CAD build for the part. Positions are in the model's coordinates, mm. A direction names the side the tool comes from. Give positions to 0.01 mm unless a question says otherwise; leave off trailing zeros. Loops run counter-clockwise (first coordinate to the right, second up) from the corner with the lowest first, then second, coordinate; pieces in that order, holes last. Notation, with made-up numbers: M 38,-18 L 65,-18 A27 ccw 65,7 Z; hole C 19.25,6 d6. An arc over 180 degrees is marked long. Answer as CSV lines item,"result".
```python
from build123d import *

# Parameters (mm, degrees)
BOSS_EXTRUDE1_DEPTH = 2.5
CUT_EXTRUDE1_DEPTH  = 2.5
SKETCH7_R           = 1.5
CUT_EXTRUDE3_DEPTH  = 2.5
SKETCH10_R          = 2.075
CUT_EXTRUDE6_DEPTH  = 2.5


with BuildPart() as part:
    # Sketch1 → Boss-Extrude1 (new body)
    with BuildSketch(Plane(origin=(0, 0, 0), x_dir=(1, 0, 0), z_dir=(0, 1, 0))):
        Polygon((0, 23.132168933), (-13.596747752, 18.714317784), (-22, 7.148233317), (-22, -7.148233317), (-13.596747752, -18.714317784), (0, -23.132168933), (13.596747752, -18.714317784), (22, -7.148233317), (22, 7.148233317), (13.596747752, 18.714317784), align=None)
    extrude(amount=BOSS_EXTRUDE1_DEPTH)

    # Sketch2 → Cut-Extrude1 (cut)
    with BuildSketch(Plane(origin=(0, 2.5, 0), x_dir=(1, 0, 0), z_dir=(0, 1, 0))):
        Polygon((0, 23.132168933), (-3.35, 22.043687951), (-3.35, 15.343687951), (3.35, 15.343687951), (3.35, 22.043687951), align=None)
        Polygon((11.729000424, 10.444223713), (15.667161615, 15.864637576), (13.596747752, 18.714317784), (10.246747752, 19.802798766), (6.308586562, 14.382384904), align=None)
        Polygon((15.627921341, 1.555421004), (22, 3.625834866), (22, 7.148233317), (19.929586138, 9.997913525), (13.557507479, 7.927499663), align=None)
        Polygon((13.557507479, -7.927499663), (19.929586138, -9.997913525), (22, -7.148233317), (22, -3.625834866), (15.627921341, -1.555421004), align=None)
        Polygon((6.308586562, -14.382384904), (10.246747752, -19.802798766), (13.596747752, -18.714317784), (15.667161615, -15.864637576), (11.729000424, -10.444223713), align=None)
        Polygon((-3.35, -15.343687951), (-3.35, -22.043687951), (0, -23.132168933), (3.35, -22.043687951), (3.35, -15.343687951), align=None)
        Polygon((-11.729000424, -10.444223713), (-15.667161615, -15.864637576), (-13.596747752, -18.714317784), (-10.246747752, -19.802798766), (-6.308586562, -14.382384904), align=None)
        Polygon((-15.627921341, -1.555421004), (-22, -3.625834866), (-22, -7.148233317), (-19.929586138, -9.997913525), (-13.557507479, -7.927499663), align=None)
        Polygon((-13.557507479, 7.927499663), (-19.929586138, 9.997913525), (-22, 7.148233317), (-22, 3.625834866), (-15.627921341, 1.555421004), align=None)
        Polygon((-6.308586562, 14.382384904), (-10.246747752, 19.802798766), (-13.596747752, 18.714317784), (-15.667161615, 15.864637576), (-11.729000424, 10.444223713), align=None)
    extrude(amount=-CUT_EXTRUDE1_DEPTH, mode=Mode.SUBTRACT)

    # Sketch7 → Cut-Extrude3 (cut)
    with BuildSketch(Plane(origin=(0, 2.5, 0), x_dir=(1, 0, 0), z_dir=(0, 1, 0))):
        with Locations(Location((0, 10, 0), (0, 0, 270))):
            Circle(SKETCH7_R)
        with Locations(Location((10, 0, 0), (0, 0, 270))):
            Circle(SKETCH7_R)
        with Locations(Location((0, -10, 0), (0, 0, 270))):
            Circle(SKETCH7_R)
        with Locations(Location((-10, 0, 0), (0, 0, 270))):
            Circle(SKETCH7_R)
    extrude(amount=-CUT_EXTRUDE3_DEPTH, mode=Mode.SUBTRACT)

    # Sketch10 → Cut-Extrude6 (cut)
    with BuildSketch(Plane(origin=(0, 2.5, 0), x_dir=(1, 0, 0), z_dir=(0, 1, 0))):
        with Locations(Location((0, 0, 0), (0, 0, 270))):
            Circle(SKETCH10_R)
    extrude(amount=-CUT_EXTRUDE6_DEPTH, mode=Mode.SUBTRACT)


solid = part.part
```
Q1. Cut at A-A (x = 0). Write the cut outline in (y, z) (3 decimals).
Solution:
outline,"M 0,-15.344 L 2.5,-15.344 L 2.5,-11.5 L 0,-11.5 Z; M 0,-8.5 L 2.5,-8.5 L 2.5,-2.075 L 0,-2.075 Z; M 0,2.075 L 2.5,2.075 L 2.5,8.5 L 0,8.5 Z; M 0,11.5 L 2.5,11.5 L 2.5,15.344 L 0,15.344 Z"
Q2. Wall check: line 1 (X direction, y = 1.05, z = 0) (3 decimals); line 2 (Z direction, x = 16, y = 0.7); line 3 (Z direction, x = -17.5, y = 1.3). Give the ranges that are in metal, low to high. Write a range as [from, to].
Solution:
line 1,"x = [-22, -11.5], [-8.5, -2.075], [2.075, 8.5], [11.5, 22]"
line 2,"z = [-15.41, -8.72], [-1.68, 1.68], [8.72, 15.41]"
line 3,"z = [-13.34, -9.21], [-2.16, 2.16], [9.21, 13.34]"
Q3. Cut at B-B (z = 0). Write the cut outline in (x, y) (3 decimals).
Solution:
outline,"M -22,0 L -11.5,0 L -11.5,2.5 L -22,2.5 Z; M -8.5,0 L -2.075,0 L -2.075,2.5 L -8.5,2.5 Z; M 2.075,0 L 8.5,0 L 8.5,2.5 L 2.075,2.5 Z; M 11.5,0 L 22,0 L 22,2.5 L 11.5,2.5 Z"
Q4. Cut at C-C (z = -18.5). Write the cut outline in (x, y), and give its area (3 significant figures).
Solution:
outline,"M -9.3,0 L -3.35,0 L -3.35,2.5 L -9.3,2.5 Z; M 3.35,0 L 9.3,0 L 9.3,2.5 L 3.35,2.5 Z"
area,"29.8 mm²"
Q5. Cut at D-D (x = 19). Write the cut outline in (y, z), and give its area (3 significant figures).
Solution:
outline,"M 0,-11.28 L 2.5,-11.28 L 2.5,-9.7 L 0,-9.7 Z; M 0,-2.65 L 2.5,-2.65 L 2.5,2.65 L 0,2.65 Z; M 0,9.7 L 2.5,9.7 L 2.5,11.28 L 0,11.28 Z"
area,"21.2 mm²"
Q6. Pin check, flat tips, straight feed: P1, Ø0.8, axis at y = 1.5, z = 20, coming from the -X side; P2, Ø1, axis at x = 5, y = 0.5, coming from the -Z side; P3, Ø0.8, axis at y = 1.5, z = -20, coming from the +X side; P4, Ø3.5, axis at x = 10, z = 0, coming from the -Y side. Stop position of each tip, or through.
Solution:
P1,"stops at x = -10.25"
P2,"stops at z = -21.67"
P3,"stops at x = 10.25"
P4,"stops at y = 0"
Q7. Mould opens along X. For faces 4 (the flat face through (-16.7, 1.27, -8.95)), 5 (the flat face through (5, 2.5, 0)), 6 (the cylindrical face through (-1.26, 1.27, -1.65)) say: released by +X, released by -X, zero draft, split by the parting line, or undercut.
Solution:
face 4,"released by -X"
face 5,"zero draft"
face 6,"undercut"
Q8. Which spindle directions (+Z, -Z, +X, -X, +Y, -Y) get a long thin tool onto all of the face, cutting with end or side? Do faces 1 (the flat face through (-13.671, 1.268, 13.116)), 2 (the flat face through (-18.859, 1.268, -2.605)), 3 (the flat face through (16.7, 1.27, 8.95)). Say none if no direction does.
Solution:
face 1,"+Z, +Y, -Y"
face 2,"+Y, -Y"
face 3,"+X, +Y, -Y"
